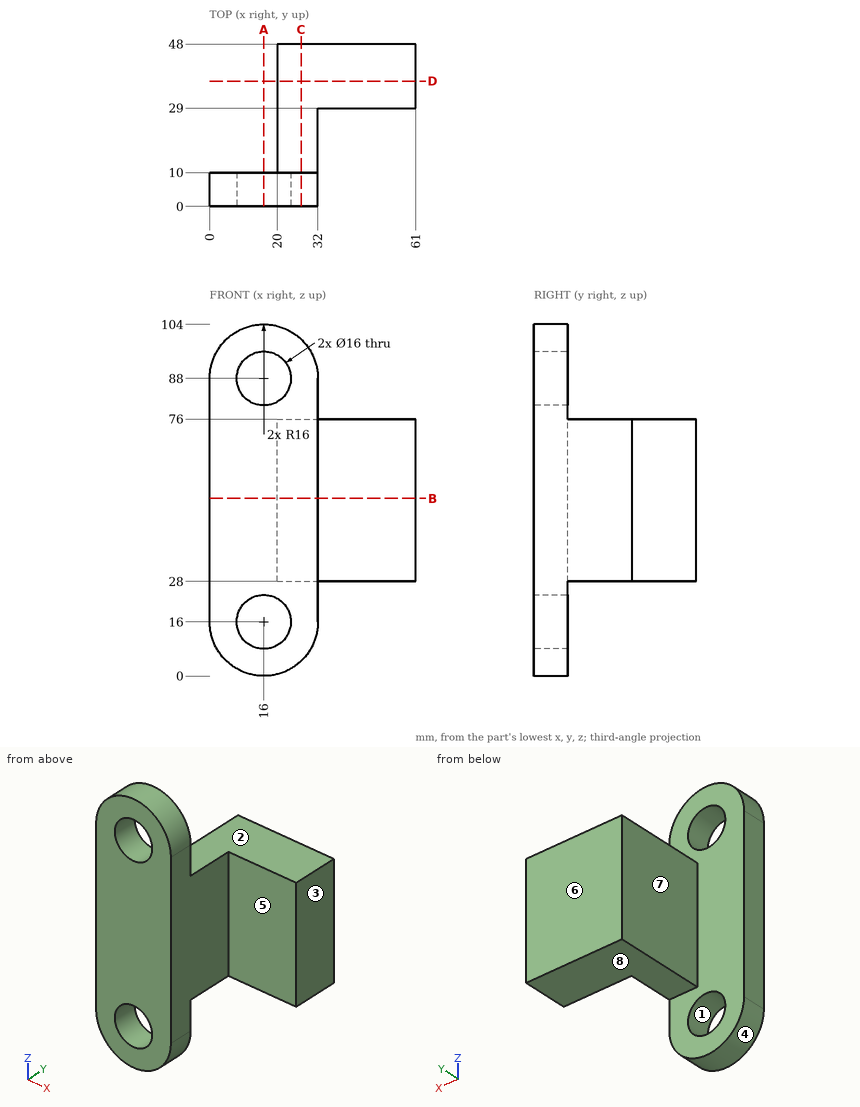
Geometry: see drawing. Coordinates: mm, zero at the bounding-box minimum. A direction names the side the tool comes from. Round coordinates to 2 decimals unless told otherwise and drop trailing zeros. Order: outer loops, then holes, each group sorted by start corner. A loop starts at its lowest first (then second) coordinate and runs counter-clockwise, first axis right, second up. Notation, with made-up numbers: (34, 17) - (69, 17) arc R13 ccw to (69, 33) - close; hole circle Ø1 at (-6.5, 27.5). An arc over 180 degrees is marked (long way). Use a Markdown table: item, result. Add a question column.
1. First-contact query: pin 1 (4 mm diameter, centred on x = 29, y = 7, fed in from -Z); pin 2 (16 mm diameter, centred on x = 16.5, z = 59.5, fed in from +Y); pin 3 (23 mm diameter, centred on x = 48.5, z = 47, fed in from -Y); pin 4 (11.5 mm diameter, centred on x = 31.5, y = 33, fed in from -Z). Flat tips, straight axial feed; report the tip coordinate or a pass-through.
2. Line query: probe 1 along X at (y, z) = (4, 88); probe 2 along Z at (x, y) = (22, 6); probe 3 along Y at (x, z) = (19.5, 36). Output: solid intervals per line, ascending.
3. Set-up query: the marked faces 4, 5, 6, 7 and 8. Return all of +Z, -Z, +X, -X, +Y, -Y with unobstructed straight access to the full face (end or side cutting, diameter ignored); none if empty.
4. Section query A-A (x = 16). Return the cut outline in (y, z).
5. Section query D-D (y = 37). Return the cut outline in (x, z), then the cut area to 3 significant figures.
6. Section query C-C (x = 27). Return the cut outline in (y, z), then the cut area to 3 significant figures.
7. Section query B-B (z = 52.5). Return the cut outline in (x, y), then the cut area to 3 significant figures.
8. Mould query, pull axis Z, two halves, no side actions, for the marked faces 1, 2 and 3. Classes: +Z half, -Z half, draft (parallel to the pull), parting line (faces both ways), or undercut.
Derived:
| question | item | result |
|---|---|---|
| 1 | pin 1 | z = 4.38 |
| 1 | pin 2 | y = 48 |
| 1 | pin 3 | y = 29 |
| 1 | pin 4 | z = 28 |
| 2 | probe 1 | 0 to 8, 24 to 32 |
| 2 | probe 2 | 1.17 to 10.71, 21.29 to 82.71, 93.29 to 102.83 |
| 2 | probe 3 | 0 to 10 |
| 3 | face 4 | -Z, +Y, -Y |
| 3 | face 5 | +Z, -Z, +X, -Y |
| 3 | face 6 | +Z, -Z, +X, -X, +Y |
| 3 | face 7 | +Z, -Z, -X, +Y |
| 3 | face 8 | -Z, +X, -X, +Y |
| 4 | outline | (0, 0) - (10, 0) - (10, 8) - (0, 8) - close; (0, 24) - (10, 24) - (10, 80) - (0, 80) - close; (0, 96) - (10, 96) - (10, 104) - (0, 104) - close |
| 5 | outline | (20, 28) - (61, 28) - (61, 76) - (20, 76) - close |
| 5 | area | 1,970 mm2 |
| 6 | outline | (0, 4.38) - (10, 4.38) - (10, 28) - (48, 28) - (48, 76) - (10, 76) - (10, 99.62) - (0, 99.62) - close |
| 6 | area | 2,780 mm2 |
| 7 | outline | (0, 0) - (32, 0) - (32, 29) - (61, 29) - (61, 48) - (20, 48) - (20, 10) - (0, 10) - close |
| 7 | area | 1,330 mm2 |
| 8 | face 1 | undercut |
| 8 | face 2 | +Z half |
| 8 | face 3 | draft |
